Geometry check sheet. Reference: the model listing, model coordinates, mm. Face numbers are marked on the shaded views. Round coordinates to 2 decimals unless told otherwise and drop trailing zeros. Loops run counter-clockwise (first coordinate to the right, second up) from the corner with the lowest first, then second, coordinate; pieces in that order, holes last. Notation, with made-up numbers: (53.5, 57) -> (97.5, 57) arc R21 ccw to (97.5, 66) -> close; hole circle Ø10 at (80, -19.75). An arc over 180 degrees is marked (long way). Use one line per item in the form item = value.
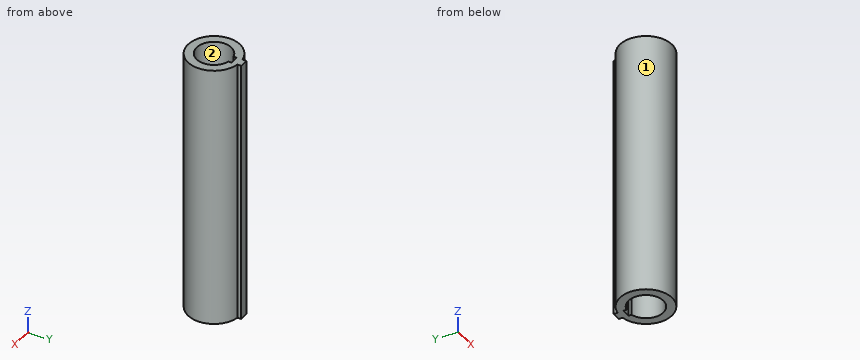
from build123d import *

# Parameters (mm, degrees)
BOSS_EXTRUDE1_DEPTH = 152.4


with BuildPart() as part:
    # Sketch1 → Boss-Extrude1 (new body)
    with BuildSketch(Plane.XY):
        with BuildLine():
            Line((-2.5, 14.790199458), (-2.5, 17))
            Line((-2.5, 17), (2.5, 17))
            Line((2.5, 17), (2.5, 14.790199458))
            ThreePointArc((2.5, 14.790199458), (0, -15), (-2.5, 14.790199458))
        make_face()
        with BuildLine():
            Line((-2.5, 9.682458366), (-2.5, 11.43))
            Line((-2.5, 11.43), (2.5, 11.43))
            Line((2.5, 11.43), (2.5, 9.682458366))
            ThreePointArc((2.5, 9.682458366), (0, -10), (-2.5, 9.682458366))
        make_face(mode=Mode.SUBTRACT)
    extrude(amount=BOSS_EXTRUDE1_DEPTH)


solid = part.part
1. Section check A-A (x = 0). Record the boundary of the cut face in (y, z), then the cut area to 3 significant figures.
Return value:
outline = (-15, 0) -> (-10, 0) -> (-10, 152.4) -> (-15, 152.4) -> close; (11.43, 0) -> (17, 0) -> (17, 152.4) -> (11.43, 152.4) -> close
area = 1,610 mm2
2. Section check B-B (y = 0). Record the boundary of the cut face in (x, z).
Return value:
outline = (-15, 0) -> (-10, 0) -> (-10, 152.4) -> (-15, 152.4) -> close; (10, 0) -> (15, 0) -> (15, 152.4) -> (10, 152.4) -> close
3. Gauge pin test, flat ends, axial feed: pin 1 (5 mm diameter, centred on x = -6.5, z = 72.5, fed in from +Y); pin 2 (1.5 mm diameter, centred on x = -6, z = 37.5, fed in from +Y); pin 3 (0.7 mm diameter, centred on y = 16, z = 86.5, fed in from +X); pin 4 (10 mm diameter, centred on x = -2, y = 1.5, fed in from +Z). Record the tip position at first contact, or that the pin passes through.
Return value:
pin_1 = 14.46
pin_2 = 14.05
pin_3 = 2.5
pin_4 = through
4. Section check C-C (z = 111). Record the boundary of the cut face in (x, y), then the cut area to 3 significant figures.
Return value:
outline = (-2.5, 14.79) arc R15 ccw (long way) to (2.5, 14.79) -> (2.5, 17) -> (-2.5, 17) -> close; hole (-2.5, 9.68) arc R10 ccw (long way) to (2.5, 9.68) -> (2.5, 11.43) -> (-2.5, 11.43) -> close
area = 395 mm2
5. Mould release check, pull along X, two halves, no side actions. Record for the marked faces 1 and 2: released by +X, released by -X, zero draft, split by the parting line, or undercut.
Return value:
face_1 = split by the parting line
face_2 = undercut
6. Material ranges on line 1 along Y through (x, z) = (0, 93.5); line 2 along X through (y, z) = (0, 39); line 3 along Y through (x, z) = (-7, 49), recorded low to high.
Return value:
line_1 = -15 to -10, 11.43 to 17
line_2 = -15 to -10, 10 to 15
line_3 = -13.27 to -7.14, 7.14 to 13.27
7. Section check D-D (y = -12.5). Record the boundary of the cut face in (x, z).
Return value:
outline = (-8.29, 0) -> (8.29, 0) -> (8.29, 152.4) -> (-8.29, 152.4) -> close
